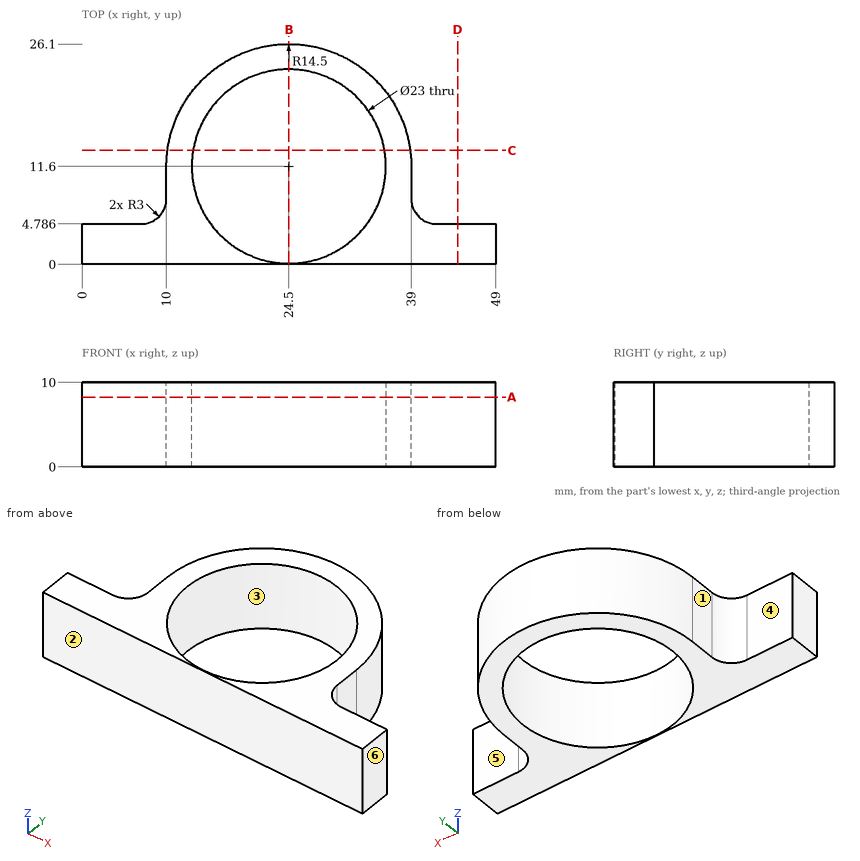
Verification items for this drawing (mm, ordinates from the low corner). A direction names the side the tool comes from. Coordinates: 2 decimals unless noted, no trailing zeros. Write each loop counter-clockwise with the first axis right and the second up, starting at its lowest first coordinate (ties: lowest second). Pieces come first, ordered by that corner, then holes. Notation, with made-up numbers: (57.5, -2) -> (107.5, -2) arc R14 cw to (107.5, 14) -> close; hole circle Ø5 at (55.25, 45.5). An arc over 180 degrees is marked (long way). One line per item, written item: value. Start each with the question number.
Q1. Thickness scan on L1, parallel to X at y = 11.75, z = 2.25; L2, parallel to X at y = 9.75, z = 1.25; L3, parallel to Y at x = 44, z = 7.25. Record the ranges inside material, lowest first. Write a range as from..to.
Q2. Cross-section at D-D on x = 44.5. Enter the section's corners in (y, z), and give its area (3 significant figures).
Q3. Go/stop test with flat-tipped pins: P1, Ø2, axis at y = 9, z = 1, coming from the -X side; P2, Ø1.5, axis at y = 19.5, z = 7, coming from the +X side; P3, Ø5.5, axis at x = 47, z = 3, coming from the +Y side; P4, Ø3, axis at x = 7.5, y = 8, coming from the +Z side. Record where each tip stops, or that it passes through.
Q4. Cross-section at B-B on x = 24.5. Enter the section's corners in (y, z).
Q5. Cross-section at C-C on y = 13.5. Enter the section's corners in (x, z) (3 decimals).
Q6. Access from +Z, -Z, +X, -X, +Y, -Y to the whole of each face (thin tool, end or side, straight path). Record for the marked faces 4, 5 and 6.
Q7. Cross-section at A-A on z = 8.25. Enter the section's corners in (x, y), and give its area (3 significant figures).
Q8. Mould release check, pull along X, two halves, no side actions. Record for the marked faces 1, 2 and 3: pulls with the +X half, pulls with the -X half, needs draft (parallel to the pull), parting line crosses it, or undercut.
Checked values:
1. L1: x = 10..13, 36..39
1. L2: x = 10..13.15, 35.85..39
1. L3: y = 0..4.79
2. outline: (0, 0) -> (4.79, 0) -> (4.79, 10) -> (0, 10) -> close
2. area: 47.9 mm²
3. P1: stops at x = 10
3. P2: stops at x = 37.11
3. P3: stops at y = 4.79
3. P4: passes through
4. outline: (0, 0) -> (0.1, 0) -> (0.1, 10) -> (0, 10) -> close; (23.1, 0) -> (26.1, 0) -> (26.1, 10) -> (23.1, 10) -> close
5. outline: (10.125, 0) -> (13.158, 0) -> (13.158, 10) -> (10.125, 10) -> close; (35.842, 0) -> (38.875, 0) -> (38.875, 10) -> (35.842, 10) -> close
6. face 4: +Z, -Z, -X, +Y
6. face 5: +Z, -Z, +X, +Y
6. face 6: +Z, -Z, +X, +Y, -Y
7. outline: (0, 0) -> (49, 0) -> (49, 4.79) -> (42, 4.79) arc R3 cw to (39, 7.79) -> (39, 11.6) arc R14.5 ccw to (10, 11.6) -> (10, 7.79) arc R3 cw to (7, 4.79) -> (0, 4.79) -> close; hole circle Ø23 at (24.5, 11.6)
7. area: 351 mm²
8. face 1: pulls with the -X half
8. face 2: needs draft
8. face 3: undercut
